```python
from build123d import *

# Parameters (mm, degrees)
SKETCH1_R               = 45
SKETCH1_R_2             = 44
BOSS_EXTRUDE1_DEPTH     = 18
BOSS_EXTRUDE2_START     = -2
SKETCH1_2_R             = 45
SKETCH1_2_R_2           = 44
BOSS_EXTRUDE2_DEPTH     = 2
M3_5X0_6_TAPPED_HOLE1_D = 2.9
CIRPATTERN1_COUNT       = 4


with BuildPart() as part:
    # Sketch1 → Boss-Extrude1 (new body)
    with BuildSketch(Plane.XY):
        Circle(SKETCH1_R)
        Circle(SKETCH1_R_2, mode=Mode.SUBTRACT)
    extrude(amount=BOSS_EXTRUDE1_DEPTH)

    # Sketch1<2> → Boss-Extrude2 (add)
    # profile 1 of 2: a face of its own
    with BuildSketch(Plane.XY.offset(BOSS_EXTRUDE2_START)):
        Circle(SKETCH1_2_R)
        Circle(SKETCH1_2_R_2, mode=Mode.SUBTRACT)
    # profile 2 of 2: a face of its own
    with BuildSketch(Plane.XY.offset(BOSS_EXTRUDE2_START)):
        Circle(SKETCH1_2_R_2)
    extrude(amount=BOSS_EXTRUDE2_DEPTH)

    # M3.5x0.6 Tapped Hole1 (through all)
    with Locations(Plane(origin=(0, 0, -2), x_dir=(-1, 0, 0), z_dir=(0, 0, -1))):
        with Locations((10.960155108, 10.960155108)):
            m3_5x0_6_tapped_hole1 = Hole(M3_5X0_6_TAPPED_HOLE1_D / 2)

    # CirPattern1: M3.5x0.6 Tapped Hole1 ×4 about axis
    cirpattern1_axis = Axis((0.011391445, -0.011391445, 0), (0, 0, 1))
    for i in range(1, CIRPATTERN1_COUNT):
        add(m3_5x0_6_tapped_hole1.rotate(cirpattern1_axis, i * 360 / CIRPATTERN1_COUNT), mode=Mode.SUBTRACT)


solid = part.part
```
Could you check a few things on this model? Use its own coordinates, in mm. A direction names the side the tool comes from. Round coordinates to 2 decimals unless told otherwise and drop trailing zeros. Loops run counter-clockwise (first coordinate to the right, second up) from the corner with the lowest first, then second, coordinate; pieces in that order, holes last. Notation, with made-up numbers: M 73.25,-21.5 L 117.25,-21.5 A27 cw 117.25,10.5 Z; hole C -35.5,54.5 d1. An arc over 180 degrees is marked long. Put each result on its own line as item: value.
Q1. On a 3-axis mill with a long thin cutter (end or side, diameter ignored), from which of +Z, -Z, +X, -X, +Y, -Y can I reach the whole of each face in a straight line? I mean faces 4 (the face through (10.43, 9.62, -0.99)), 5 (the face through (-1, 1, 0)). Say none if no direction works.
Check result:
face 4: +Z, -Z
face 5: +Z
Q2. Thinking about a two-plate mould opening in X: for faces 1 (the face through (20.765, -39.923, 7.86)), 2 (the face through (-1, 1, -2)), 3 (the face through (12.43, -11.05, -0.99)), which applies, released by +X, released by -X, zero draft, split by the parting line, or undercut?
Check result:
face 1: split by the parting line
face 2: zero draft
face 3: undercut
Q3. For pin 1 (2.5 mm diameter, centred on x = -10.96, y = 10.96, fed in from -Z); pin 2 (4.5 mm diameter, centred on x = 10.98, y = 10.96, fed in from +Z); pin 3 (6 mm diameter, centred on y = -10, z = 11, fed in from +X); pin 4 (1.5 mm diameter, centred on y = -7.5, z = 9, fed in from -X), each with a flat end and sliding along its axis, tell me the tip position at first contact or that it passes through.
Check result:
pin 1: through
pin 2: z = 0
pin 3: x = 44.45
pin 4: x = -44.49
Q4. I need wall thicknesses on probe 1 along Y at (x, z) = (0, 5); probe 2 along Z at (x, y) = (-13, 2.5); probe 3 along Y at (x, z) = (12, 6). Which ranges of each line are inside material? Lowest first, please.
Check result:
probe 1: -45 to -44, 44 to 45
probe 2: -2 to 0
probe 3: -43.37 to -42.33, 42.33 to 43.37
Q5. Imagine slicing it at B-B (z = 6.75). Write out the boundary of the cut face in (x, y).
Check result:
outline: C 0,0 d90; hole C 0,0 d88
Q6. Imagine slicing it at C-C (x = -33). Write out the boundary of the cut face in (y, z), then the cut area to 3 significant figures.
Check result:
outline: M -30.59,-2 L 30.59,-2 L 30.59,18 L 29.1,18 L 29.1,0 L -29.1,0 L -29.1,18 L -30.59,18 Z
area: 176 mm2
Q7. Imagine slicing it at A-A (y = 0). Write out the boundary of the cut face in (x, z).
Check result:
outline: M -45,-2 L 45,-2 L 45,18 L 44,18 L 44,0 L -44,0 L -44,18 L -45,18 Z
